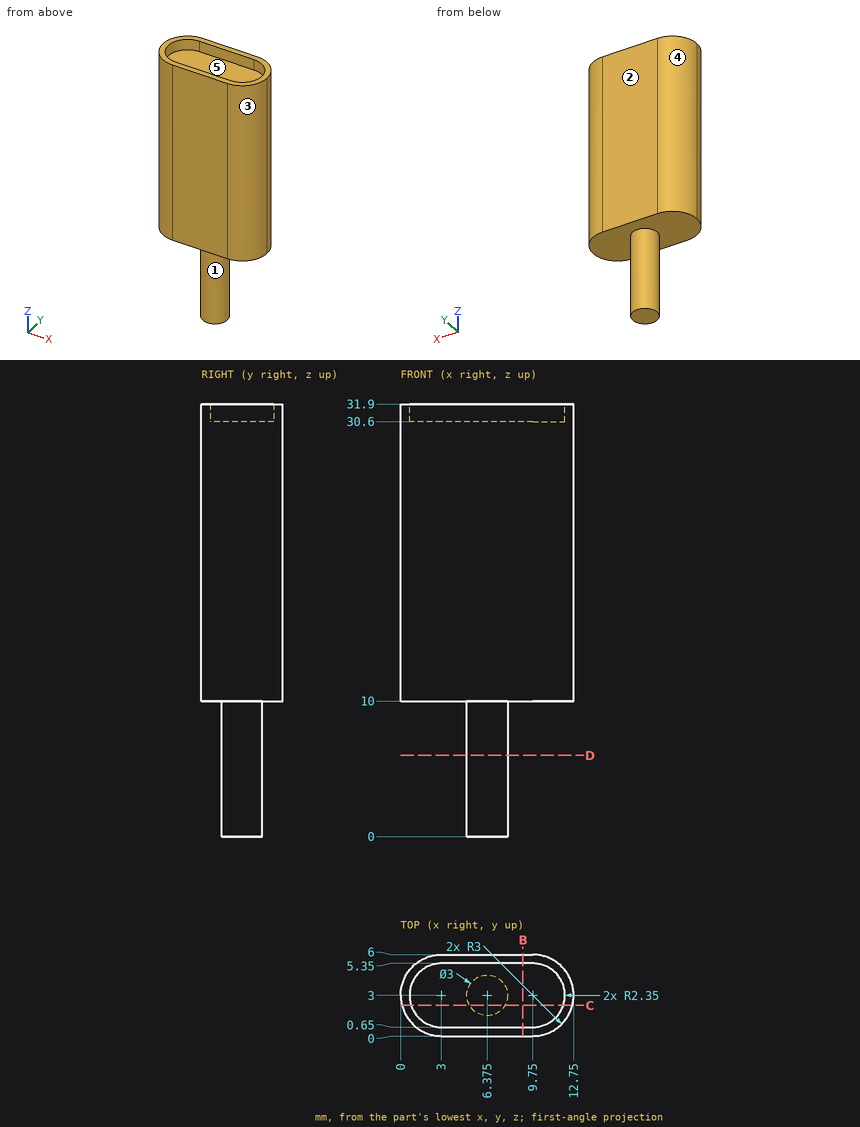
Input: dimensioned drawing with shaded views. Units: mm. Origin: part minimum x, y, z. A direction names the side the tool comes from. Give positions to 0.01 mm unless a question says otherwise; leave off trailing zeros. Loops run counter-clockwise (first coordinate to the right, second up) from the corner with the lowest first, then second, coordinate; pieces in that order, holes last. Notation, with made-up numbers: M 85.5,47.5 L 139.5,47.5 A20 cw 139.5,63.5 Z; hole C 12.25,-17.5 d5. An arc over 180 degrees is marked long. Put each result on its own line as item: value.
1) Material intervals for L1, parallel to Z at x = 10.5, y = 3; L2, parallel to Z at x = 12.25, y = 4.5; L3, parallel to Y at x = 10.75, z = 11.5, sorted ascending. Write a range as from..to.
Computed values:
L1: z = 10..30.6
L2: z = 10..31.9
L3: y = 0.17..5.83
2) Mould query, pull axis X, two halves, no side actions, for the marked faces 3, 4 and 5. Classes: released by +X, released by -X, zero draft, split by the parting line, or undercut.
Computed values:
face 3: released by +X
face 4: released by -X
face 5: undercut
3) Cut plane D-D, the plane z = 6. Return the cut outline in (x, y) (3 decimals).
Computed values:
outline: C 6.375,3 d3
4) Reachability of the marked faces 1 and 2 from +Z, -Z, +X, -X, +Y, -Y: full face, straight path, thin tool, end or side. Return the list, or none.
Computed values:
face 1: -Z
face 2: +Z, -Z, +X, -X, +Y
5) Cut plane C-C, the plane y = 2.25. Return the cut outline in (x, z).
Computed values:
outline: M 0.1,10 L 5.08,10 L 5.08,0 L 7.67,0 L 7.67,10 L 12.65,10 L 12.65,31.9 L 11.98,31.9 L 11.98,30.6 L 0.77,30.6 L 0.77,31.9 L 0.1,31.9 Z
6) First-contact query: P1, Ø0.7, axis at x = 7.5, z = 31, coming from the -Y side; P2, Ø2, axis at y = 5.5, z = 25.5, coming from the -X side; P3, Ø1.5, axis at y = 4.5, z = 25, coming from the +X side. Flat tips, straight axial feed; report the tip coordinate or a pass-through.
Computed values:
P1: stops at y = 0
P2: stops at x = 0.4
P3: stops at x = 12.65
7) Cut plane B-B, the plane x = 9. Return the cut outline in (y, z).
Computed values:
outline: M 0,10 L 6,10 L 6,31.9 L 5.35,31.9 L 5.35,30.6 L 0.65,30.6 L 0.65,31.9 L 0,31.9 Z
